Geometry: final body of the model. Coordinates: model frame, mm. A direction names the side the tool comes from. Give positions to 0.01 mm unless a question says otherwise; leave off trailing zeros. Order: outer loops, then holes, each group sorted by start corner. A loop starts at its lowest first (then second) coordinate and runs counter-clockwise, first axis right, second up. Notation, with made-up numbers: M -11.75,43 L 44.25,43 A28 cw 44.25,78 Z; hole C 79,-8.75 d6. An arc over 180 degrees is marked long. Use CSV: the item, a comma, the result in double quotes.
```python
from build123d import *


with BuildPart() as f1:
    # F0 (on Front) → F1 (revolve)
    with BuildSketch(Plane.XZ):
        with BuildLine():
            Line((2.44, 0), (1.54, 0))
            Line((1.54, 0), (1.54, -2))
            Line((1.54, -2), (0, -2))
            Line((0, -2), (0, -10.36))
            Line((0, -10.36), (2.405, -10.36))
            Line((2.405, -10.36), (2.405, -11.57))
            Line((2.405, -11.57), (3.305, -11.57))
            Line((3.305, -11.57), (3.305, -10.36))
            ThreePointArc((3.305, -10.36), (4.542437, -9.847437), (5.055, -8.61))
            Line((5.055, -8.61), (5.055, -3.75))
            ThreePointArc((5.055, -3.75), (4.542437, -2.512563), (3.305, -2))
            Line((3.305, -2), (2.44, -2))
            Line((2.44, -2), (2.44, 0))
        make_face()
    revolve(axis=Axis((0, 0, 28.045654), (0, 0, 1)))


solid = f1.part
```
1. Section A-A, the plane y = 0. Return the cut outline in (x, z) (3 decimals).
Answer:
outline,"M -5.055,-8.61 A1.75 ccw -3.305,-10.36 L -3.305,-11.57 L -2.405,-11.57 L -2.405,-10.36 L 2.405,-10.36 L 2.405,-11.57 L 3.305,-11.57 L 3.305,-10.36 A1.75 ccw 5.055,-8.61 L 5.055,-3.75 A1.75 ccw 3.305,-2 L 2.44,-2 L 2.44,0 L 1.54,0 L 1.54,-2 L -1.54,-2 L -1.54,0 L -2.44,0 L -2.44,-2 L -3.305,-2 A1.75 ccw -5.055,-3.75 Z"
2. Section C-C, the plane z = -5.5. Return the cut outline in (x, y) (3 decimals).
Answer:
outline,"C 0,0 d10.11"
3. Pin query (flat end, axial travel): pin 1 Ø4 at (x, y) = (0, 0) entering from -Z; pin 2 Ø2 at (y, z) = (3.5, -4.5) entering from -X; pin 3 Ø1.5 at (x, y) = (3, -3.5) entering from +Z. Return the tip coordinate at first contact, or that it passes through.
Answer:
pin 1,"z = -10.36"
pin 2,"x = -4.39"
pin 3,"z = -2.09"
4. Reachability of faces 1 (the face through (-1.22, -0.94, -1.01)), 2 (the face through (0, 0, -10.36)) from +Z, -Z, +X, -X, +Y, -Y: full face, straight path, thin tool, end or side. Return the list, or none.
Answer:
face 1,"+Z"
face 2,"-Z"
5. Line query: line 1 (Y direction, x = 0, z = -11.25) (3 decimals); line 2 (Y direction, x = 0, z = -0.35); line 3 (Z direction, x = -0.75, y = 0.25). Output: solid intervals per line, ascending.
Answer:
line 1,"-3.305 to -2.405, 2.405 to 3.305"
line 2,"-2.44 to -1.54, 1.54 to 2.44"
line 3,"-10.36 to -2"
6. Pull-direction query (Y, two-part tool) for faces 3 (the face through (-4.01, -3.08, -6.15)), 4 (the face through (0, -2, 0)), 5 (the face through (0, 0, -2)), 6 (the face through (-2.403, 0.106, -10.973)); classes: +Y half, -Y half, draft (parallel to the pull), parting line (faces both ways), or undercut.
Answer:
face 3,"parting line"
face 4,"draft"
face 5,"undercut"
face 6,"undercut"
